```python
from build123d import *

# Parameters (mm, degrees)
SKETCH1_W           = 3.5
SKETCH1_H           = 3.5
SKETCH1_R           = 1
BOSS_EXTRUDE1_DEPTH = 18
CHAMFER1_SIZE       = 0.5


with BuildPart() as part:
    # Sketch1 → Boss-Extrude1 (new body)
    with BuildSketch(Plane(origin=(0, 0, 0), x_dir=(1, 0, 0), z_dir=(0, 1, 0))):
        Rectangle(SKETCH1_W, SKETCH1_H)
        Circle(SKETCH1_R, mode=Mode.SUBTRACT)
    extrude(amount=BOSS_EXTRUDE1_DEPTH)

    # Chamfer1
    chamfer1_edges = [part.edges().sort_by_distance(p)[0] for p in [
        (1.75, 9, 1.75),
        (-1.75, 9, 1.75),
        (-1.75, 9, -1.75),
        (1.75, 9, -1.75),
    ]]
    chamfer(chamfer1_edges, length=CHAMFER1_SIZE)


solid = part.part
```
Source: CAD feature listing. Evaluate the final solid. Frame: model axes, mm. Coordinates: 2 decimals unless noted, no trailing zeros. Write each loop counter-clockwise with the first axis right and the second up, starting at its lowest first coordinate (ties: lowest second). Pieces come first, ordered by that corner, then holes. Notation, with made-up numbers: M 38.5,-25.75 L 77.5,-25.75 A11 cw 77.5,-15.75 Z; hole C 15,53.25 d2. An arc over 180 degrees is marked long. Answer as a JSON object with one key per item and string values.
1. Cut plane B-B on x = 0. Output: boundary loops of the cut face in (y, z).
Evaluation:
{"outline": "M 0,-1.75 L 18,-1.75 L 18,-1 L 0,-1 Z; M 0,1 L 18,1 L 18,1.75 L 0,1.75 Z"}
2. Draft query along X for faces 1 (the cylindrical face through (0, 9, 1)), 2 (the flat face through (-1.75, 9, 0)), 3 (the flat face through (-1, 0, 1)). Return one class per face: released by +X, released by -X, zero draft, split by the parting line, or undercut.
Evaluation:
{"face 1": "undercut", "face 2": "released by -X", "face 3": "zero draft"}
3. Cut plane C-C on y = 14.75. Output: boundary loops of the cut face in (x, z).
Evaluation:
{"outline": "M -1.75,-1.25 L -1.25,-1.75 L 1.25,-1.75 L 1.75,-1.25 L 1.75,1.25 L 1.25,1.75 L -1.25,1.75 L -1.75,1.25 Z; hole C 0,0 d2"}
4. Ray query, L1, parallel to X at y = 12, z = 0; L2, parallel to Z at x = -0.2, y = 13.75; L3, parallel to Z at x = 0.7, y = 4. Return the intervals inside material, ascending.
Evaluation:
{"L1": "-1.75 to -1, 1 to 1.75", "L2": "-1.75 to -0.98, 0.98 to 1.75", "L3": "-1.75 to -0.71, 0.71 to 1.75"}
5. Cut plane A-A on z = 0. Output: boundary loops of the cut face in (x, y).
Evaluation:
{"outline": "M -1.75,0 L -1,0 L -1,18 L -1.75,18 Z; M 1,0 L 1.75,0 L 1.75,18 L 1,18 Z"}
6. Cut plane D-D on z = 1.45. Output: boundary loops of the cut face in (x, y).
Evaluation:
{"outline": "M -1.55,0 L 1.55,0 L 1.55,18 L -1.55,18 Z"}
